Here's how the part is built. I have some questions about the finished solid (model axes, mm). Face numbers are marked on the shaded views. Give positions to 0.01 mm unless a question says otherwise; leave off trailing zeros. Write each loop counter-clockwise with the first axis right and the second up, starting at its lowest first coordinate (ties: lowest second). Pieces come first, ordered by that corner, then holes. Notation, with made-up numbers: M -37,82.5 L 0,82.5 A13 ccw 0,91.5 Z; hole C 27.25,-13 d8. An arc over 180 degrees is marked long. Use one line per item in the form item = value. Start each with the question number.
from build123d import *

# Parameters (mm, degrees)
BOSS_EXTRUDE1_DEPTH = 10
SKETCH2_R           = 2.5
CUT_EXTRUDE1_DEPTH  = 10
SKETCH3_R           = 1.5
CUT_EXTRUDE2_DEPTH  = 10
SKETCH6_R           = 1.5
CUT_EXTRUDE3_DEPTH  = 10
SKETCH7_W           = 10
SKETCH7_H           = 10
CUT_EXTRUDE4_DEPTH  = 4


with BuildPart() as part:
    # Sketch1 → Boss-Extrude1 (new body)
    with BuildSketch(Plane(origin=(0, 0, 0), x_dir=(1, 0, 0), z_dir=(0, 1, 0))):
        Polygon((-79, 100), (-79, 79), (-100, 79), (-100, -79), (-79, -79), (-79, -100), (79, -100), (79, -79), (100, -79), (100, 79), (79, 79), (79, 100), align=None)
    extrude(amount=BOSS_EXTRUDE1_DEPTH)

    # Sketch2 → Cut-Extrude1 (cut)
    with BuildSketch(Plane(origin=(0, 10, 0), x_dir=(1, 0, 0), z_dir=(0, 1, 0))):
        with Locations(Location((-90, 0, 0), (0, 0, 270))):
            Circle(SKETCH2_R)
        with Locations(Location((90, 0, 0), (0, 0, 90))):
            Circle(SKETCH2_R)
    extrude(amount=-CUT_EXTRUDE1_DEPTH, mode=Mode.SUBTRACT)

    # Sketch3 → Cut-Extrude2 (cut)
    with BuildSketch(Plane(origin=(0, 10, 0), x_dir=(1, 0, 0), z_dir=(0, 1, 0))):
        with Locations(Location((27.9, 83.74, 0), (0, 0, 270))):
            Circle(SKETCH3_R)
        with Locations(Location((27.9, 5, 0), (0, 0, 270))):
            Circle(SKETCH3_R)
        with Locations(Location((-27.9, 5, 0), (0, 0, 90))):
            Circle(SKETCH3_R)
        with Locations(Location((-27.9, 83.74, 0), (0, 0, 90))):
            Circle(SKETCH3_R)
        with Locations(Location((-27.9, -5, 0), (0, 0, 270))):
            Circle(SKETCH3_R)
        with Locations(Location((27.9, -5, 0), (0, 0, 90))):
            Circle(SKETCH3_R)
        with Locations(Location((27.9, -83.74, 0), (0, 0, 90))):
            Circle(SKETCH3_R)
        with Locations(Location((-27.9, -83.74, 0), (0, 0, 270))):
            Circle(SKETCH3_R)
    extrude(amount=-CUT_EXTRUDE2_DEPTH, mode=Mode.SUBTRACT)

    # Sketch6 → Cut-Extrude3 (cut)
    with BuildSketch(Plane(origin=(0, 10, 0), x_dir=(1, 0, 0), z_dir=(0, 1, 0))):
        with Locations(Location((-37.54, 25.4, 0), (0, 0, 270))):
            Circle(SKETCH6_R)
        with Locations(Location((-52.78, -25.4, 0), (0, 0, 270))):
            Circle(SKETCH6_R)
        with Locations(Location((-80.27, -25.4, 0), (0, 0, 270))):
            Circle(SKETCH6_R)
    extrude(amount=-CUT_EXTRUDE3_DEPTH, mode=Mode.SUBTRACT)

    # Sketch7 → Cut-Extrude4 (cut)
    with BuildSketch(Plane(origin=(0, 10, 0), x_dir=(1, 0, 0), z_dir=(0, 1, 0))):
        with Locations((-90, 0)):
            Rectangle(SKETCH7_W, SKETCH7_H)
        with Locations((90, 0)):
            Rectangle(SKETCH7_W, SKETCH7_H)
    extrude(amount=-CUT_EXTRUDE4_DEPTH, mode=Mode.SUBTRACT)


solid = part.part
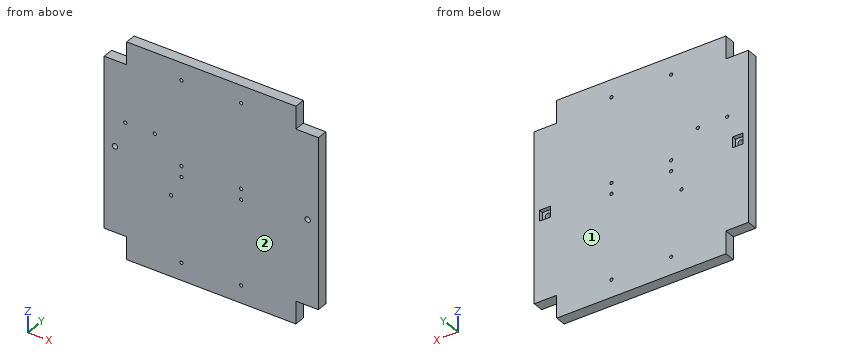
1) Suppose I cut it at A-A, the plane x = -90. List the corners of the cut face in (y, z) for me.
2) Suppose I cut it at B-B, the plane y = 4. State how many separate pieces and enclosed holes the cut face has, and give its area (3 significant figures).
3) Thinking about a two-plate mould opening in Y: for the marked faces 1 and 2, which applies, released by +Y, released by -Y, zero draft, split by the parting line, or undercut?
4) Will these pins go through, and if not, where does the flat tip stop? P1, Ø3, axis at x = -94.5, y = 6.5, coming from the +Z side; P2, Ø5, axis at y = 6.5, z = 91, coming from the -X side.
5) Please list where these lines run through material, in increasing order: line 1 (X direction, y = 3, z = -5); line 2 (X direction, y = 2.5, z = -83.74); line 3 (Z direction, x = -80, y = 1.75).
Checks:
q1.outline = M 0,-79 L 10,-79 L 10,-5 L 6,-5 L 6,-2.5 L 0,-2.5 Z; M 0,2.5 L 6,2.5 L 6,5 L 10,5 L 10,79 L 0,79 Z
q2.separate_pieces = 1
q2.enclosed_holes = 13
q2.area = 38,100 mm^2
q3.face_1 = released by +Y
q3.face_2 = released by -Y
q4.P1 = 79
q4.P2 = -79
q5.line_1 = -100 to -29.4, -26.4 to 26.4, 29.4 to 100
q5.line_2 = -79 to -29.4, -26.4 to 26.4, 29.4 to 79
q5.line_3 = -79 to 23.92, 26.88 to 79
